Part model, mm, in its own coordinate system. Face numbers are marked on the shaded views. A direction names the side the tool comes from. Coordinates: 2 decimals unless noted, no trailing zeros. Loops run counter-clockwise (first coordinate to the right, second up) from the corner with the lowest first, then second, coordinate; pieces in that order, holes last. Notation, with made-up numbers: M -30,81.25 L 13,81.25 A17 cw 13,97.25 Z; hole C 5,41.5 d4. An arc over 180 degrees is marked long. Answer as a JSON object with one key per item and string values. Group by question number.
1. Drop flat-ended pins along their axis: pin 1 Ø16.5 at (x, y) = (9.5, 32) entering from +Z (3 decimals); pin 2 Ø18.5 at (y, z) = (-1, 9.5) entering from +X (3 decimals); pin 3 Ø15.5 at (x, z) = (14, 36.5) entering from +Y; pin 4 Ø15.5 at (x, z) = (51.5, 26.5) entering from -Y. Give the stop position or say it passes through.
2. Saw through at C-C on x = 66.5. Write the cut outline in (y, z) (3 decimals), then the cut area to 3 significant figures.
3. Drill centre lines: L1, parallel to Z at x = 40, y = -26 (3 decimals); L2, parallel to Z at x = 95, y = 2 (3 decimals); L3, parallel to X at y = -12, z = 15.5 (3 decimals). Where is each one in solid material? Low to high.
4. Saw through at B-B on y = 31.5. Write the cut outline in (x, z) (3 decimals).
5. Saw through at A-A on z = 3. Write the cut outline in (x, y) (3 decimals).
6. Saw through at D-D on x = 99.5. Write the cut outline in (y, z) (3 decimals), then the cut area to 3 significant figures.
7. 3-axis set-ups, long thin cutter, end or side, ignore diameter. For the marked faces 1, 2, 3 and 4: which of +Z, -Z, +X, -X, +Y, -Y reach the whole face in a straight line?
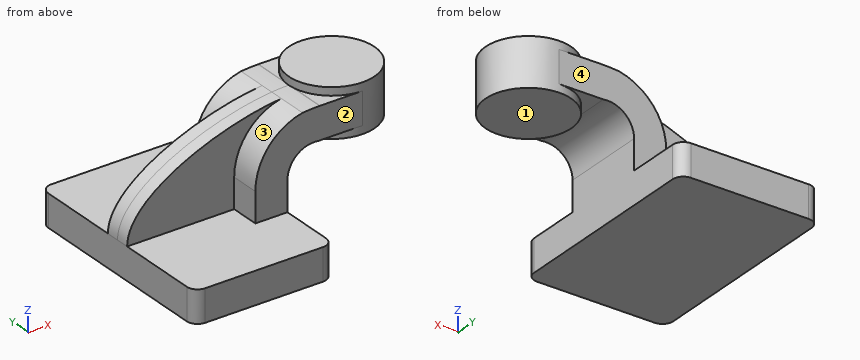
from build123d import *

# Parameters (mm, degrees)
F1_DEPTH = 63.5
F2_DEPTH = 25.4
F3_DEPTH = 7.9375
F5_R     = 6.35


with BuildPart() as f1:
    # F0 (on Front) → F1 (new body, symmetric)
    with BuildSketch(Plane.XZ):
        Polygon((22.225, 9.525), (-41.275, 9.525), (-41.275, -9.525), (41.275, -9.525), (41.275, 9.525), align=None)
    extrude(amount=F1_DEPTH, both=True)

    # F0 (on Front) → F2 (join, symmetric)
    with BuildSketch(Plane.XZ):
        with BuildLine():
            Line((22.225, 27.176042), (22.225, 9.525))
            Line((22.225, 9.525), (41.275, 9.525))
            Line((41.275, 9.525), (41.275, 27.176042))
            ThreePointArc((41.275, 27.176042), (46.791196, 39.205623), (59.506283, 42.8752))
            Line((59.506283, 42.8752), (60.325, 42.8752))
            Line((60.325, 42.8752), (60.325, 61.924634))
            add(Edge.make_bspline(
                [(50.225098, 61.407626), (53.729785, 61.737464), (57.113469, 61.913471), (60.325, 61.924634)],
                knots=[104.739527, 104.739527, 104.739527, 104.739527, 114.283242, 114.283242, 114.283242, 114.283242], degree=3))
            ThreePointArc((50.225098, 61.407626), (30.116615, 49.288295), (22.225, 27.176042))
        make_face()
        with BuildLine():
            add(Edge.make_bspline(
                [(60.325, 61.924634), (60.43361, 61.925011), (60.542023, 61.9252), (60.650237, 61.9252)],
                knots=[114.283242, 114.283242, 114.283242, 114.283242, 114.605999, 114.605999, 114.605999, 114.605999], degree=3))
            Line((60.325, 61.924634), (60.325, 42.8752))
            Line((60.325, 42.8752), (85.725, 42.8752))
            Line((85.725, 42.8752), (85.725, 61.9252))
            Line((85.725, 61.9252), (60.650237, 61.9252))
        make_face()
    extrude(amount=F2_DEPTH, both=True)

    # F0 (on Front) → F3 (join, symmetric)
    with BuildSketch(Plane.XZ):
        with BuildLine():
            add(Edge.make_bspline(
                [(-41.275, 9.525), (-41.275, 35.639968), (11.762158, 57.787757), (50.225098, 61.407626)],
                knots=[0, 0, 0, 0, 104.739527, 104.739527, 104.739527, 104.739527], degree=3))
            Line((-41.275, 9.525), (22.225, 9.525))
            Line((22.225, 9.525), (22.225, 27.176042))
            ThreePointArc((22.225, 27.176042), (30.116615, 49.288295), (50.225098, 61.407626))
        make_face()
    extrude(amount=F3_DEPTH, both=True)

    # F0 (on Front) → F4 (revolve)
    with BuildSketch(Plane.XZ):
        Polygon((111.125, 66.675), (85.725, 66.675), (85.725, 61.9252), (85.725, 42.8752), (85.725, 38.1), (111.125, 38.1), align=None)
    revolve(axis=Axis((85.725, 0, 52.3875), (0, 0, 1)))

    # F5
    f5_edges = [f1.edges().sort_by_distance(p)[0] for p in [
        (41.275, -63.5, 0),
        (-41.275, -63.5, 0),
        (41.275, 63.5, 0),
        (-41.275, 63.5, 0),
    ]]
    fillet(f5_edges, radius=F5_R)


solid = f1.part
Outcome:
{
 "1": {"pin 1": "stops at z = 9.525", "pin 2": "stops at x = 41.275", "pin 3": "stops at y = 7.94", "pin 4": "passes through"},
 "2": {"outline": "M -25.4,42.875 L -16.6,42.875 L -16.6,38.1 L 16.6,38.1 L 16.6,42.875 L 25.4,42.875 L 25.4,61.925 L 16.6,61.925 L 16.6,66.675 L -16.6,66.675 L -16.6,61.925 L -25.4,61.925 Z", "area": "1,280 mm²"},
 "3": {"L1": "z = -9.525 to 9.525", "L2": "z = 38.1 to 66.675", "L3": "x = 22.225 to 41.275"},
 "4": {"outline": "M -41.275,-9.525 L 41.275,-9.525 L 41.275,9.525 L -41.275,9.525 Z"},
 "5": {"outline": "M -41.275,-57.15 A6.35 ccw -34.925,-63.5 L 34.925,-63.5 A6.35 ccw 41.275,-57.15 L 41.275,57.15 A6.35 ccw 34.925,63.5 L -34.925,63.5 A6.35 ccw -41.275,57.15 Z"},
 "6": {"outline": "M -21.34,38.1 L 21.34,38.1 L 21.34,66.675 L -21.34,66.675 Z", "area": "1,220 mm²"},
 "7": {"face 1": "-Z, +X, +Y, -Y", "face 2": "+Z, +X, -X, -Y", "face 3": "+Z, -X, -Y", "face 4": "+Z, +X, -X, +Y"}
}
